Geometry check sheet. Reference: the model listing, model coordinates, mm. Face numbers are marked on the shaded views. Coordinates: 2 decimals unless noted, no trailing zeros. Write each loop counter-clockwise with the first axis right and the second up, starting at its lowest first coordinate (ties: lowest second). Pieces come first, ordered by that corner, then holes. Notation, with made-up numbers: M 55,46.5 L 72,46.5 A5 cw 72,55.5 Z; hole C 40,56 d5. An arc over 180 degrees is marked long. Answer as a JSON object with one key per item and string values. Group by question number.
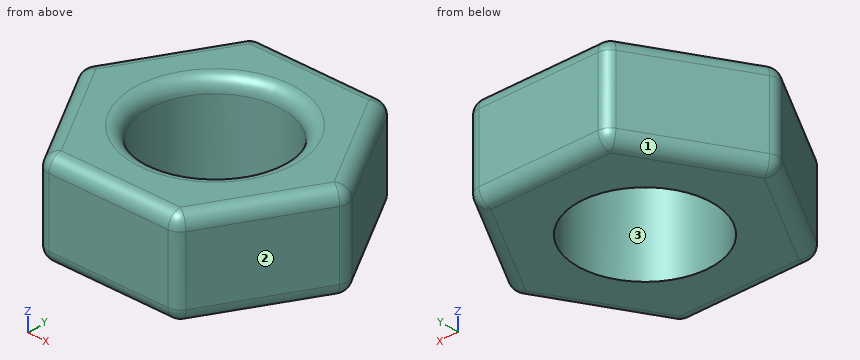
```python
from build123d import *

# Parameters (mm, degrees)
SKETCH1_R           = 5
BOSS_EXTRUDE1_DEPTH = 7
FILLET1_R           = 1
FILLET2_R           = 1


with BuildPart() as part:
    # Sketch1 → Boss-Extrude1 (new body)
    with BuildSketch(Plane.XY):
        Polygon((10, 0), (5, 8.660254038), (-5, 8.660254038), (-10, 0), (-5, -8.660254038), (5, -8.660254038), align=None)
        Circle(SKETCH1_R, mode=Mode.SUBTRACT)
    extrude(amount=BOSS_EXTRUDE1_DEPTH)

    # Fillet1
    fillet1_edges = [part.edges().sort_by_distance(p)[0] for p in [
        (5, -8.660254038, 3.5),
        (-5, -8.660254038, 3.5),
        (-10, 0, 3.5),
        (-5, 8.660254038, 3.5),
        (5, 8.660254038, 3.5),
        (10, 0, 3.5),
        (-5, 0, 7),
    ]]
    fillet(fillet1_edges, radius=FILLET1_R)

    # Fillet2
    fillet2_edges = [part.edges().sort_by_distance(p)[0] for p in [
        (7.5, -4.330127019, 7),
        (7.5, 4.330127019, 7),
        (0, 8.660254038, 7),
        (-7.5, 4.330127019, 7),
        (-7.5, -4.330127019, 7),
        (0, -8.660254038, 7),
        (4.922649731, 8.526279442, 7),
        (-4.922649731, 8.526279442, 7),
        (-9.845299462, 0, 7),
        (-4.922649731, -8.526279442, 7),
        (4.922649731, -8.526279442, 7),
        (9.845299462, 0, 7),
        (7.5, 4.330127019, 0),
        (7.5, -4.330127019, 0),
        (0, -8.660254038, 0),
        (-7.5, -4.330127019, 0),
        (-7.5, 4.330127019, 0),
        (0, 8.660254038, 0),
        (4.922649731, 8.526279442, 0),
        (-4.922649731, 8.526279442, 0),
        (-9.845299462, 0, 0),
        (-4.922649731, -8.526279442, 0),
        (4.922649731, -8.526279442, 0),
        (9.845299462, 0, 0),
    ]]
    fillet(fillet2_edges, radius=FILLET2_R)


solid = part.part
```
1) Go/stop test with flat-tipped pins: pin 1 Ø1.5 at (y, z) = (6, 5.5) entering from +X; pin 2 Ø1.5 at (y, z) = (4, 3) entering from -X. Record where each tip stops, or that it passes through.
2) Section check B-B (z = 4.5). Record the cut outline in (x, y), then the cut area to 3 significant figures.
3) Material ranges on probe 1 along Y at (x, z) = (0, 4.7); probe 2 along X at (y, z) = (-1.25, 1.5); probe 3 along Y at (x, z) = (-4.5, 0.5), recorded low to high. Write a range as [from, to].
4) Section check C-C (z = 0.5). Record the cut outline in (x, y), then the cut area to 3 significant figures.
5) Section check A-A (x = 0). Record the cut outline in (y, z).
6) Draft check along X on the marked faces 1, 2 and 3. Enter one of: +X half, -X half, draft (parallel to the pull), parting line (faces both ways), or undercut.
Entries:
{
 "1": {"pin 1": "x = 6.97", "pin 2": "x = -8.12"},
 "2": {"outline": "M -9.71,-0.5 L -5.29,-8.16 A1 ccw -4.42,-8.66 L 4.42,-8.66 A1 ccw 5.29,-8.16 L 9.71,-0.5 A1 ccw 9.71,0.5 L 5.29,8.16 A1 ccw 4.42,8.66 L -4.42,8.66 A1 ccw -5.29,8.16 L -9.71,0.5 A1 ccw Z; hole C 0,0 d10", "area": "181 mm^2"},
 "3": {"probe 1": "[-8.66, -5], [5, 8.66]", "probe 2": "[-9.28, -4.84], [4.84, 9.28]", "probe 3": "[-8.52, -2.18], [2.18, 8.52]"},
 "4": {"outline": "M -9.6,-0.43 L -5.17,-8.09 A0.87 ccw -4.42,-8.53 L 4.42,-8.53 A0.87 ccw 5.17,-8.09 L 9.6,-0.43 A0.87 ccw 9.6,0.43 L 5.17,8.09 A0.87 ccw 4.42,8.53 L -4.42,8.53 A0.87 ccw -5.17,8.09 L -9.6,0.43 A0.87 ccw Z; hole C 0,0 d10", "area": "173 mm^2"},
 "5": {"outline": "M -8.66,1 A1 ccw -7.66,0 L -5,0 L -5,6 A1 ccw -6,7 L -7.66,7 A1 ccw -8.66,6 Z; M 5,0 L 7.66,0 A1 ccw 8.66,1 L 8.66,6 A1 ccw 7.66,7 L 6,7 A1 ccw 5,6 Z"},
 "6": {"face 1": "-X half", "face 2": "+X half", "face 3": "undercut"}
}
